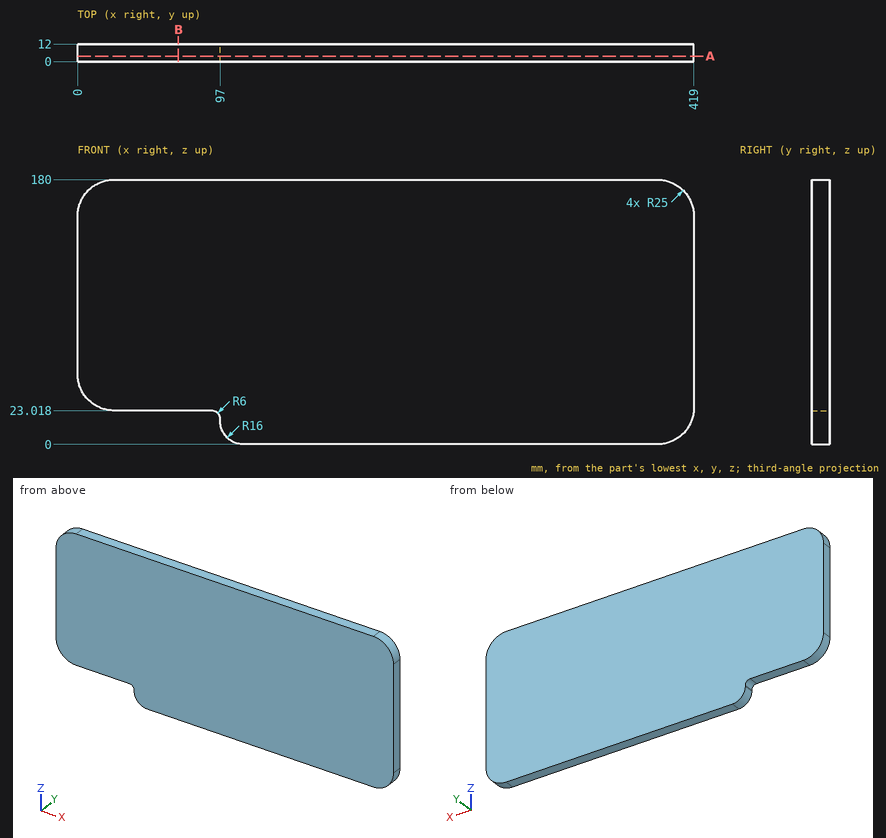
Design review of the part shown in the three views and the two pictorial views. Dimensions are in mm from the part's minimum x, y and z. Give positions to 0.01 mm unless a question says otherwise; leave off trailing zeros. Loops run counter-clockwise (first coordinate to the right, second up) from the corner with the lowest first, then second, coordinate; pieces in that order, holes last. Notation, with made-up numbers: (-13, 1) - (15, 1) arc R17 ccw to (15, 30) - close; hole circle Ø4 at (-13, 27). An arc over 180 degrees is marked (long way). Use CSV: the item, a comma, the result in double quotes. Start each with the question number.
1. Insertion check: P1, Ø3, axis at x = 340, y = 2.5, coming from the -Z side; P2, Ø0.8, axis at y = 5, z = 16.5, coming from the -X side. Each pin has a flat end and moves straight along its axis. Give the tip position at first contact, or say it passes through.
2. Wall thickness on L1, parallel to X at y = 7.75, z = 17; L2, parallel to X at y = 9.25, z = 16: over which ranges is each line inside the solid? List them lowest first.
3. Add section B-B (x = 68.5). State the section outline as (y, z) points.
4. Add section A-A (y = 3.75). State the section outline as (x, z) points, plus the area to 3 significant figures.
Results found:
1,P1,"stops at z = 0"
1,P2,"stops at x = 97"
2,L1,"x = 97 to 417.69"
2,L2,"x = 97 to 417.32"
3,outline,"(0, 23.02) - (12, 23.02) - (12, 180) - (0, 180) - close"
4,outline,"(0, 48.02) arc R25 ccw to (25, 23.02) - (91, 23.02) arc R6 cw to (97, 17.02) - (97, 16) arc R16 ccw to (113, 0) - (394, 0) arc R25 ccw to (419, 25) - (419, 155) arc R25 ccw to (394, 180) - (25, 180) arc R25 ccw to (0, 155) - close"
4,area,"72,600 mm²"
